from build123d import *

# Parameters (mm, degrees)
BOSS_EXTRUDE2_DEPTH = 4
BOSS_EXTRUDE3_START = 4
BOSS_EXTRUDE3_DEPTH = 4
CUT_EXTRUDE1_DEPTH  = 4
SKETCH7_R           = 1
CUT_EXTRUDE2_DEPTH  = 51.104291233
SKETCH9_R           = 1
CUT_EXTRUDE8_DEPTH  = 51.58102411
FILLET1_R           = 10
FILLET2_R           = 10
FILLET3_R           = 3


with BuildPart() as part:
    # Sketch1 → Boss-Extrude2 (new body)
    with BuildSketch(Plane(origin=(0, 0, 0), x_dir=(1, 0, 0), z_dir=(0, 1, 0))):
        with BuildLine():
            Line((-20, 2), (20, 13.8))
            Line((20, 13.8), (42.1, 13.8))
            ThreePointArc((42.1, 13.8), (48, 7.9), (42.1, 2))
            Line((42.1, 2), (20, 2))
            Line((20, 2), (20, -2))
            Line((20, -2), (-20, -2))
            Line((-20, -2), (-20, 2))
        make_face()
    extrude(amount=BOSS_EXTRUDE2_DEPTH)

    # Sketch4 → Boss-Extrude3 (add)
    with BuildSketch(Plane(origin=(0, 0, 0), x_dir=(-1, 0, 0), z_dir=(0, -1, 0)).offset(BOSS_EXTRUDE3_START)):
        with BuildLine():
            Line((-20, 2), (-42.1, 2))
            ThreePointArc((-42.1, 2), (-48, 7.9), (-42.1, 13.8))
            Line((-42.1, 13.8), (-20, 13.8))
            Line((-20, 13.8), (-20, 2))
        make_face()
    extrude(amount=-BOSS_EXTRUDE3_DEPTH)

    # Sketch6 → Cut-Extrude1 (cut)
    with BuildSketch(Plane.XZ.offset(4)):
        with BuildLine():
            Line((39.899748285, -4.9), (27.981348848, -5.907102203))
            ThreePointArc((27.981348848, -5.907102203), (25.988451051, -7.9), (27.981348848, -9.892897797))
            Line((27.981348848, -9.892897797), (39.867781655, -10.876291126))
            ThreePointArc((39.867781655, -10.876291126), (45.820310688, -7.919899599), (39.899748285, -4.9))
        make_face()
    extrude(amount=-CUT_EXTRUDE1_DEPTH, mode=Mode.SUBTRACT)

    # Sketch7 → Cut-Extrude2 (cut, through all)
    with BuildSketch(Plane.XZ):
        with Locations(Location((42.1, -7.9, 0), (0, 0, 270))):
            Circle(SKETCH7_R)
    extrude(amount=-CUT_EXTRUDE2_DEPTH, mode=Mode.SUBTRACT)

    # Sketch9 → Cut-Extrude8 (cut, through all)
    with BuildSketch(Plane(origin=(0, 4, 0), x_dir=(1, 0, 0), z_dir=(0, 1, 0))):
        with Locations(Location((-14.5, 0, 0), (0, 0, 270))):
            Circle(SKETCH9_R)
        with Locations(Location((14.5, 0, 0), (0, 0, 270))):
            Circle(SKETCH9_R)
    extrude(amount=-CUT_EXTRUDE8_DEPTH, mode=Mode.SUBTRACT)

    # Fillet1
    # the kernel refuses this fillet: 10 mm, written as the material it takes off along each edge
    with BuildSketch(Plane(origin=(20, -4, -33.8), x_dir=(1, 0, 0), z_dir=(0, 0, 1))) as fillet1_piece_1:
        with BuildLine():
            CenterArc((8, 10), FILLET1_R, 216.869897646, 53.130102354)
            Line((0, 4), (-0.16, 3.88))
            ThreePointArc((-0.16, 3.88), (-0.2, 2), (-0.2, 0))
            Line((-0.2, 0), (0, -0.2))
            Line((0, -0.2), (8, -0.2))
            Line((8, -0.2), (8, 0))
        make_face()
    extrude(amount=51.8, mode=Mode.SUBTRACT)

    # Fillet2
    fillet2_edges = [part.edges().sort_by_distance(p)[0] for p in [
        (20, 2, -13.8),
    ]]
    fillet(fillet2_edges, radius=FILLET2_R)

    # Fillet3
    fillet3_edges = [part.edges().sort_by_distance(p)[0] for p in [
        (-20, 4, 0),
        (20, 4, 0),
    ]]
    fillet(fillet3_edges, radius=FILLET3_R)


solid = part.part
Here's how the part is built. I have some questions about the finished solid (model axes, mm). A direction names the side the tool comes from. Coordinates: 2 decimals unless noted, no trailing zeros. Loops run counter-clockwise (first coordinate to the right, second up) from the corner with the lowest first, then second, coordinate; pieces in that order, holes last. Notation, with made-up numbers: (-5, 26.5) -> (3, 26.5) arc R20 cw to (3, 43.5) -> close; hole circle Ø2 at (58.25, -16.5). An arc over 180 degrees is marked (long way). Use one line per item in the form item = value. Start each with the question number.
(1) If we section it at A-A (z = 0): Please give me the cut outline in (x, y).
(2) On a 3-axis mill with a long thin cutter (end or side, diameter ignored), from which of +Z, -Z, +X, -X, +Y, -Y can I reach the whole of each face in a straight line? I mean faces 4 (the face through (5, 0, -4)), 5 (the face through (45.82, -2.03, -8.03)), 6 (the face through (0, 2, 2)), 7 (the face through (19.1, 3.14, 0.03)), 8 (the face through (-19.1, 3.14, 0.07)). Say none if no direction works.
(3) If we section it at C-C (y = -2.75): Please give me the cut outline in (x, z).
(4) If we section it at B-B (x = 14.5): Please give me the cut outline in (y, z), then the cut area to 3 significant figures.
(5) We'd pull the mould along Z, two halves only. Please class faces 1 (the face through (16, 4, -6)), 2 (the face through (13.524, 2.028, -0.217)), 3 (the face through (32, 0, -2)): pulls with the +Z half, pulls with the -Z half, needs draft (parallel to the pull), parting line crosses it, or undercut.
(6) If we section it at D-D (z = -7.9): Please give me the cut outline in (x, y).
(7) Please list where these lines run through material, in increasing order: line 1 along X through (y, z) = (1.5, 0); line 2 along X through (y, z) = (3, 0); line 3 along Y through (x, z) = (43, -4.75).
(8) Will these pins go through, and if not, where does the flat tip stop? pin 1 (1 mm diameter, centred on x = 21.5, y = 3, fed in from +Z); pin 2 (1.6 mm diameter, centred on x = 14.5, z = 0, fed in from +Y); pin 3 (4.5 mm diameter, centred on x = 42.1, z = -7.9, fed in from -Y); pin 4 (4 mm diameter, centred on y = -1, z = -1, fed in from +X).
Verdict:
q1.outline = (-20, 0) -> (-15.5, 0) -> (-15.5, 4) -> (-17, 4) arc R3 ccw to (-20, 1) -> close; (-13.5, 0) -> (13.5, 0) -> (13.5, 4) -> (-13.5, 4) -> close; (15.5, 0) -> (20, 0) -> (20, 1) arc R3 ccw to (17, 4) -> (15.5, 4) -> close
q2.face_4 = +Z, -Z, -X, -Y
q2.face_5 = -Y
q2.face_6 = +Z, +X, -X, +Y, -Y
q2.face_7 = +Z, +X, +Y
q2.face_8 = +Z, -Z, -X, +Y
q3.outline = (23.16, -13.8) -> (42.1, -13.8) arc R5.9 ccw to (42.1, -2) -> (23.16, -2) -> close; hole (27.98, -9.89) -> (39.87, -10.88) arc R3.72 ccw (long way) to (39.9, -4.9) -> (27.98, -5.91) arc R1.99 ccw to start
q4.outline = (0, -12.18) -> (4, -12.18) -> (4, -1) -> (0, -1) -> close; (0, 1) -> (4, 1) -> (4, 2) -> (0, 2) -> close
q4.area = 48.7 mm²
q5.face_1 = needs draft
q5.face_2 = undercut
q5.face_3 = pulls with the +Z half
q6.outline = (0, 0) -> (20, 0) arc R10 ccw to (25.99, -3.8) -> (25.99, 0) -> (41.1, 0) -> (41.1, 4) -> (0, 4) -> close; (43.1, 0) -> (45.82, 0) -> (45.82, -4) -> (48, -4) -> (48, 4) -> (43.1, 4) -> close
q7.line_1 = -19.96 to -15.5, -13.5 to 13.5, 15.5 to 19.96
q7.line_2 = -19.24 to -15.5, -13.5 to 13.5, 15.5 to 19.24
q7.line_3 = 0 to 4
q8.pin_1 = -2
q8.pin_2 = through
q8.pin_3 = 0
q8.pin_4 = 45.39
